Verification items for the finished model (mm, model axes). A direction names the side the tool comes from. Give positions to 0.01 mm unless a question says otherwise; leave off trailing zeros. Order: outer loops, then holes, each group sorted by start corner. A loop starts at its lowest first (then second) coordinate and runs counter-clockwise, first axis right, second up. Notation, with made-up numbers: (65, 1.5) -> (105, 1.5) arc R14 ccw to (105, 23.5) -> close; hole circle Ø5 at (-26.75, -38). An arc over 180 degrees is marked (long way). One line per question, with ' | ' between items. Start each with the question number.
Q1. Section check B-B on z = 2.2. Record the cut outline in (x, y) (3 decimals).
Q2. Material ranges on probe 1 along Y at (x, z) = (-9, 1.2); probe 2 along Y at (x, z) = (-6, 0.2); probe 3 along X at (y, z) = (4, 0.45), recorded low to high. Write a range as [from, to].
Q3. Mould release check, pull along Y, two halves, no side actions. Record for faces 4 (the cylindrical face through (8.12, 4.46, 1.48)), 5 (the cylindrical face through (-10.872, 2.525, 1.479)), 6 (the flat face through (0, 10, 0)): released by +Y, released by -Y, zero draft, split by the parting line, or undercut.
Q4. Go/stop test with flat-tipped pins: pin 1 (1.1 mm diameter, centred on x = 6.5, z = 1, fed in from +Y); pin 2 (0.7 mm diameter, centred on x = -7, z = 1, fed in from +Y); pin 3 (1.1 mm diameter, centred on y = 8.5, z = 2, fed in from +X). Record where each tip stops, or that it passes through.
Q5. Section check D-D on y = 4.25. Record the cut outline in (x, z).
Q6. Section check A-A on y = 8. Record the cut outline in (x, z).
Q7. Access from +Z, -Z, +X, -X, +Y, -Y to the whole of each face (thin tool, end or side, straight path). Record for faces 1 (the flat face through (0, 10, 3)), 2 (the cylindrical face through (5.93, 4.59, 1.48)), 3 (the flat face through (6, 7.5, 1)).
Q8. Section check C-C on x = 10.25. Record the cut outline in (y, z), plus the area to 3 significant figures.
from build123d import *

# Parameters (mm, degrees)
ESQUISSE1_R        = 1.5
BOSS_EXTRU_2_DEPTH = 3


with BuildPart() as part:
    # Esquisse1 → Boss.-Extru.2 (new body)
    with BuildSketch(Plane.XY):
        with BuildLine():
            Line((5.230618988, 7.5), (7.5, 7.5))
            Line((7.5, 7.5), (7.5, 8.9))
            Line((7.5, 8.9), (-7.5, 8.9))
            Line((-7.5, 8.9), (-7.5, 7.5))
            Line((-7.5, 7.5), (-5.230618988, 7.5))
            Line((-5.230618988, 7.5), (-5.230618988, 5.375))
            ThreePointArc((-5.230618988, 5.375), (-5.918936429, 4.606103727), (-6.495190528, 3.75))
            ThreePointArc((-6.495190528, 3.75), (-10.934773091, 2.560417438), (-12.124355653, 7))
            ThreePointArc((-12.124355653, 7), (-9.780131311, 10.017436376), (-6.707371512, 12.288660114))
            ThreePointArc((-6.707371512, 12.288660114), (-4.47014813, 12.872261577), (-2.411034891, 11.820685714))
            ThreePointArc((-2.411034891, 11.820685714), (0, 10.75), (2.411034891, 11.820685714))
            ThreePointArc((2.411034891, 11.820685714), (3.975330286, 12.779130538), (5.80943088, 12.737759334))
            ThreePointArc((5.80943088, 12.737759334), (9.414650572, 10.36167721), (12.124355653, 7))
            ThreePointArc((12.124355653, 7), (10.934773091, 2.560417438), (6.495190528, 3.75))
            ThreePointArc((6.495190528, 3.75), (5.918936429, 4.606103727), (5.230618988, 5.375))
            Line((5.230618988, 5.375), (5.230618988, 7.5))
        make_face()
        with Locations((9.309773091, 5.375)):
            Circle(ESQUISSE1_R, mode=Mode.SUBTRACT)
        with Locations((-9.309773091, 5.375)):
            Circle(ESQUISSE1_R, mode=Mode.SUBTRACT)
    extrude(amount=BOSS_EXTRU_2_DEPTH)


solid = part.part
Filled in:
1) outline: (-12.124, 7) arc R3.25 ccw to (-6.495, 3.75) arc R7.5 cw to (-5.231, 5.375) -> (-5.231, 7.5) -> (-7.5, 7.5) -> (-7.5, 8.9) -> (7.5, 8.9) -> (7.5, 7.5) -> (5.231, 7.5) -> (5.231, 5.375) arc R7.5 cw to (6.495, 3.75) arc R3.25 ccw to (12.124, 7) arc R14 ccw to (5.809, 12.738) arc R3.25 ccw to (2.411, 11.821) arc R3.25 cw to (-2.411, 11.821) arc R3.25 ccw to (-6.707, 12.289) arc R14 ccw to start; hole circle Ø3 at (-9.31, 5.375); hole circle Ø3 at (9.31, 5.375)
2) probe 1: [2.14, 3.91], [6.84, 10.72] | probe 2: [4.5, 7.5], [8.9, 12.67] | probe 3: [-12.25, -9.91], [-8.71, -6.34], [6.34, 8.71], [9.91, 12.25]
3) face 4: undercut | face 5: split by the parting line | face 6: zero draft
4) pin 1: y = 12.67 | pin 2: y = 12.33 | pin 3: x = 11.52
5) outline: (-12.36, 0) -> (-10.3, 0) -> (-10.3, 3) -> (-12.36, 3) -> close; (-8.32, 0) -> (-6.18, 0) -> (-6.18, 3) -> (-8.32, 3) -> close; (6.18, 0) -> (8.32, 0) -> (8.32, 3) -> (6.18, 3) -> close; (10.3, 0) -> (12.36, 0) -> (12.36, 3) -> (10.3, 3) -> close
6) outline: (-11.49, 0) -> (-7.5, 0) -> (-7.5, 3) -> (-11.49, 3) -> close; (7.5, 0) -> (11.49, 0) -> (11.49, 3) -> (7.5, 3) -> close
7) face 1: +Z, +X, -X, +Y, -Y | face 2: +Z, -Z, -Y | face 3: +Z, -Z
8) outline: (2.26, 0) -> (4.21, 0) -> (4.21, 3) -> (2.26, 3) -> close; (6.54, 0) -> (9.54, 0) -> (9.54, 3) -> (6.54, 3) -> close | area: 14.8 mm²
